from build123d import *

# Parameters (mm, degrees)
SKETCH_1_W          = 43
SKETCH_1_H          = 7.5
EXTRUDE_1_DEPTH     = 2
SKETCH_2_R          = 1.65
CUT_EXTRUDE_2_DEPTH = 11.5
FILLET_1_R          = 3.75
SKETCH_3_W          = 30
SKETCH_3_H          = 14
EXTRUDE_3_DEPTH     = 2
SKETCH_4_W          = 15
SKETCH_4_H          = 32
EXTRUDE_4_DEPTH     = 2
SKETCH_5_R          = 2.1
CUT_EXTRUDE_3_DEPTH = 13
FILLET_3_R          = 5
FILLET_5_R          = 0.5
FILLET_6_R          = 0.5
FILLET_7_R          = 0.5


with BuildPart() as part:
    # 草圖1 → 填料-伸長1 (new body)
    with BuildSketch(Plane(origin=(0, 0, 0), x_dir=(0, 0, -1), z_dir=(1, 0, 0))):
        Rectangle(SKETCH_1_W, SKETCH_1_H)
    extrude(amount=EXTRUDE_1_DEPTH)

    # 草圖2 → 除料-伸長2 (cut)
    with BuildSketch(Plane(origin=(2, 0, 0), x_dir=(0, 0, -1), z_dir=(1, 0, 0))):
        with Locations((-18.5, 0)):
            Circle(SKETCH_2_R)
        with Locations((18.5, 0)):
            Circle(SKETCH_2_R)
    extrude(amount=-CUT_EXTRUDE_2_DEPTH, mode=Mode.SUBTRACT)

    # 圓角1
    fillet_1_edges = [part.edges().sort_by_distance(p)[0] for p in [
        (1, -3.75, -21.5),
        (1, 3.75, -21.5),
        (1, -3.75, 21.5),
        (1, 3.75, 21.5),
    ]]
    fillet(fillet_1_edges, radius=FILLET_1_R - 0.0001)  # a hair under: the kernel refuses the full size

    # 草圖3 → 填料-伸長3 (add)
    with BuildSketch(Plane.ZY):
        Rectangle(SKETCH_3_W, SKETCH_3_H)
    extrude(amount=-EXTRUDE_3_DEPTH)

    # 草圖4 → 填料-伸長4 (add)
    with BuildSketch(Plane(origin=(0, -7, 0), x_dir=(1, 0, 0), z_dir=(0, 1, 0))):
        with Locations((7.5, 0)):
            Rectangle(SKETCH_4_W, SKETCH_4_H)
    extrude(amount=EXTRUDE_4_DEPTH)

    # 草圖5 → 除料-伸長3 (cut)
    with BuildSketch(Plane(origin=(0, -5, 0), x_dir=(-1, 0, 0), z_dir=(0, 1, 0))):
        with Locations(Location((-8.4, 12, 0), (0, 0, 90))):
            Circle(SKETCH_5_R)
        with Locations(Location((-8.4, 4, 0), (0, 0, 90))):
            Circle(SKETCH_5_R)
        with Locations(Location((-8.4, -4, 0), (0, 0, 90))):
            Circle(SKETCH_5_R)
        with Locations(Location((-8.4, -12, 0), (0, 0, 90))):
            Circle(SKETCH_5_R)
    extrude(amount=-CUT_EXTRUDE_3_DEPTH, mode=Mode.SUBTRACT)

    # 圓角3
    fillet_3_edges = [part.edges().sort_by_distance(p)[0] for p in [
        (15, -6, 16),
        (15, -6, -16),
    ]]
    fillet(fillet_3_edges, radius=FILLET_3_R)

    # 圓角5
    fillet_5_edges = [part.edges().sort_by_distance(p)[0] for p in [
        (1, -3.75, -15),
        (1, -3.75, 15),
        (1, -5, -15),
        (1, -5, 15),
    ]]
    fillet(fillet_5_edges, radius=FILLET_5_R)

    # 圓角6
    fillet_6_edges = [part.edges().sort_by_distance(p)[0] for p in [
        (5, -5, 16),
        (13.535533906, -5, 14.535533906),
        (15, -5, 0),
        (13.535533906, -5, -14.535533906),
        (5, -5, -16),
    ]]
    fillet(fillet_6_edges, radius=FILLET_6_R - 0.0001)  # a hair under: the kernel refuses the full size

    # 圓角7
    fillet_7_edges = [part.edges().sort_by_distance(p)[0] for p in [
        (1, 7, 15),
        (1, 7, -15),
    ]]
    fillet(fillet_7_edges, radius=FILLET_7_R)


solid = part.part
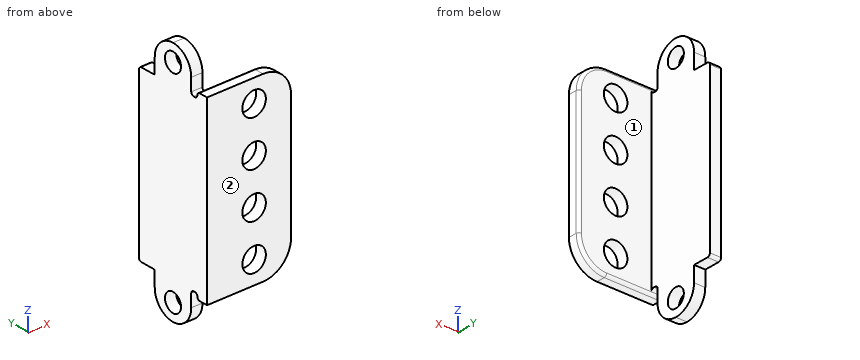
Part model, mm, in its own coordinate system. Face numbers are marked on the shaded views. A direction names the side the tool comes from. Round coordinates to 2 decimals unless told otherwise and drop trailing zeros. Order: outer loops, then holes, each group sorted by start corner. A loop starts at its lowest first (then second) coordinate and runs counter-clockwise, first axis right, second up. Notation, with made-up numbers: (-6, 33) -> (46, 33) arc R21 cw to (46, 61) -> close; hole circle Ø1 at (45.5, 85.5). An arc over 180 degrees is marked (long way). Put each result on its own line as item: value.
Q1. Tool access for the marked faces 1 and 2: list every direction of +Z, -Z, +X, -X, +Y, -Y with a clear straight run to the whole face (end or side of a thin tool).
From the geometry:
face 1: +Z, -Z, +X, +Y
face 2: +Z, -Z, +X, -X, -Y
Q2. Band-saw the part on B-B (z = -1.5). Give the cut face in (x, y).
From the geometry:
outline: (0, -7) -> (15, -7) -> (15, -5.5) arc R0.5 ccw to (14.5, -5) -> (2, -5) -> (2, 7) -> (0, 7) -> close
Q3. Band-saw the part on C-C (x = 5.25). Give the cut face in (y, z).
From the geometry:
outline: (-7, -16) -> (-5.5, -16) arc R0.5 ccw to (-5, -15.5) -> (-5, 15.5) arc R0.5 ccw to (-5.5, 16) -> (-7, 16) -> close
Q4. Pin check, flat tips, straight feed: pin 1 Ø0.6 at (x, z) = (1.5, 17) entering from -Y; pin 2 Ø1.7 at (x, y) = (4, -6.5) entering from -Z; pin 3 Ø2 at (y, z) = (0, 18.5) entering from -X; pin 4 Ø1 at (x, y) = (1, 5.5) entering from +Z. Stop position of each tip, or through.
From the geometry:
pin 1: stops at y = -3.75
pin 2: stops at z = -16
pin 3: passes through
pin 4: stops at z = 15
Q5. Band-saw the part on A-A (z = 4). Give the cut face in (x, y), and give its area (3 significant figures).
From the geometry:
outline: (0, -7) -> (6.3, -7) -> (6.3, -5) -> (2, -5) -> (2, 7) -> (0, 7) -> close; (10.5, -7) -> (15, -7) -> (15, -5.5) arc R0.5 ccw to (14.5, -5) -> (10.5, -5) -> close
area: 45.5 mm2
Q6. Band-saw the part on D-D (z = 18.5). Give the cut face in (x, y).
From the geometry:
outline: (0, -3.67) -> (2, -3.67) -> (2, -1.65) -> (0, -1.65) -> close; (0, 1.65) -> (2, 1.65) -> (2, 3.67) -> (0, 3.67) -> close
Q7. Wall check: line 1 (X direction, y = -6.1, z = -4); line 2 (Z direction, x = 1.5, y = -1.25); line 3 (X direction, y = -4, z = 7.5). Give the ranges that are in metal, low to high. Write a range as [from, to].
From the geometry:
line 1: x = [0, 6.3], [10.5, 15]
line 2: z = [-21.29, -19.58], [-17.42, 17.42], [19.58, 21.29]
line 3: x = [0, 2]
